The listing builds one solid part. Answer for the finished solid, in the listing's coordinates (mm). A direction names the side the tool comes from. Coordinates: 2 decimals unless noted, no trailing zeros. Order: outer loops, then holes, each group sorted by start corner. A loop starts at its lowest first (then second) coordinate and runs counter-clockwise, first axis right, second up. Notation, with made-up numbers: (-6, -4) - (43, -4) arc R11 ccw to (43, 16) - close; hole circle Ø3 at (-28, 54.25). An arc over 180 degrees is marked (long way). Use one line per item in the form item = value. Start each with the question number.
Item 1: Consider line 1 along X through (y, z) = (-66.3, 0); line 2 along X through (y, z) = (-68.85, 0); line 3 along X through (y, z) = (-64.5, 0). Determine where each line is inside the solid, lowest interval first. Write a range as [from, to].
Item 2: The mould has two halves that part along Z. Classify faces 1 (the flat face through (13, -66.8, -3)), 2 (the cylindrical face through (21.07, -64.93, -5.5)), 3 (the flat face through (-22.5, -65, 0)), 4 (the flat face through (2, 0, -5)): released by +Z, released by -Z, zero draft, split by the parting line, or undercut.
Item 3: Each of these flat-tipped pins is pushed along its axis until it touches: pin 1 Ø4.5 at (x, y) = (1, 0.5) entering from +Z; pin 2 Ø2 at (x, z) = (6.5, 0) entering from -Y; pin 3 Ø3 at (x, z) = (-5, -1) entering from +Y. Where does it stop, or does it pass through?
Item 4: Section A-A, the plane y = -58 is taken. Write down the section's boundary in (x, z).
Item 5: A tool of negligible diameter and unlimited length cuts with its end or side. For faces 5 (the cylindrical face through (-7.493, 0.33, -0.563)), 6 (the flat face through (-20, -60, -3)), 7 (the cylindrical face through (-21, -65.07, 5.57)), 8 (the cylindrical face through (9.63, -63.35, -1.19)), 9 (the cylindrical face through (-6.399, -67.465, 1.908)), from which of +Z, -Z, +X, -X, +Y, -Y can it reach the whole face along a straight path? Write none if from no direction.
from build123d import *

# Parameters (mm, degrees)
SKETCH_1_R                = 15
SKETCH_1_R_2              = 0.5
EXTRUDE_1_DEPTH           = 7
CUT_EXTRUDE_START         = -12
SKETCH_2_R                = 7.5
SKETCH_2_R_2              = 0.5
CUT_EXTRUDE_1_DEPTH       = 12
CHAMFER_1_SIZE            = 3
EXTRUDE_2_DEPTH           = 7
CUT_EXTRUDE_2_DEPTH       = 5
FILLET_1_R                = 5
MM_1_D                    = 4
MM_1_DEPTH                = 5
MM_1_TIP                  = 1.201721238
HOLE_WIZARD_1_D           = 6.4
HOLE_WIZARD_1_DEPTH       = 10
HOLE_WIZARD_1_CBORE_D     = 11
HOLE_WIZARD_1_CBORE_DEPTH = 6.8


with BuildPart() as part:
    # 草图1 → 凸台-拉伸1 (new, symmetric)
    with BuildSketch(Plane.XY):
        Circle(SKETCH_1_R)
        Circle(SKETCH_1_R_2, mode=Mode.SUBTRACT)
    extrude(amount=EXTRUDE_1_DEPTH, both=True)

    # 草图2 → 切除-拉伸1 (cut)
    with BuildSketch(Plane.XY.offset(7).offset(CUT_EXTRUDE_START)):
        Circle(SKETCH_2_R)
        Circle(SKETCH_2_R_2, mode=Mode.SUBTRACT)
    extrude(amount=CUT_EXTRUDE_1_DEPTH, mode=Mode.SUBTRACT)

    # 倒角1
    chamfer_1_edges = [part.edges().sort_by_distance(p)[0] for p in [
        (-7.5, 0, 7),
    ]]
    chamfer(chamfer_1_edges, length=CHAMFER_1_SIZE)

    # 草图3 → 凸台-拉伸2 (add, symmetric)
    with BuildSketch(Plane.XY):
        with BuildLine():
            Line((-22.5, -60), (-22.5, -70))
            Line((-22.5, -70), (22.5, -70))
            Line((22.5, -70), (22.5, -60))
            Line((22.5, -60), (9, -60))
            Line((9, -60), (9, -12))
            ThreePointArc((9, -12), (0, -15), (-9, -12))
            Line((-9, -12), (-9, -60))
            Line((-9, -60), (-22.5, -60))
        make_face()
    extrude(amount=EXTRUDE_2_DEPTH, both=True)

    # 草图4 → 切除-拉伸2 (cut)
    with BuildSketch(Plane.XZ.offset(70)):
        with BuildLine():
            Line((6, 2), (8, 2))
            ThreePointArc((8, 2), (10, 0), (8, -2))
            Line((8, -2), (6, -2))
            ThreePointArc((6, -2), (4, 0), (6, 2))
        make_face()
    extrude(amount=-CUT_EXTRUDE_2_DEPTH, mode=Mode.SUBTRACT)

    # 圆角1
    fillet_1_edges = [part.edges().sort_by_distance(p)[0] for p in [
        (-22.5, -65, -7),
        (22.5, -65, 7),
        (-22.5, -65, 7),
        (22.5, -65, -7),
    ]]
    fillet(fillet_1_edges, radius=FILLET_1_R)

    # 大小mm 暗销孔1
    with Locations(Plane(origin=(-7, -70, 0), x_dir=(0, 0, -1), z_dir=(0, -1, 0))):
        with Locations((0, 0)):
            Hole(MM_1_D / 2, depth=MM_1_DEPTH)
            with Locations((0, 0, -(MM_1_DEPTH + MM_1_TIP / 2))):  # 118° drill point
                Cone(0, MM_1_D / 2, MM_1_TIP, mode=Mode.SUBTRACT)

    # 打孔尺寸(%根据)内六角圆柱头螺钉的类型1
    with Locations(Plane(origin=(-15, -60, 0), x_dir=(0, 0, 1), z_dir=(0, 1, 0))):
        with Locations((0, 0), (0, 30)):
            CounterBoreHole(HOLE_WIZARD_1_D / 2, HOLE_WIZARD_1_CBORE_D / 2, HOLE_WIZARD_1_CBORE_DEPTH, depth=HOLE_WIZARD_1_DEPTH)


solid = part.part
Response:
q1.line_1 = [-22.5, -20.5], [-9.5, -9], [-5, 4], [20.5, 22.5]
q1.line_2 = [-22.5, -18.2], [-11.8, -9], [-5, 4], [10, 11.8], [18.2, 22.5]
q1.line_3 = [-22.5, -20.5], [-9.5, -8.17], [-5.83, 9.5], [20.5, 22.5]
q2.face_1 = undercut
q2.face_2 = released by -Z
q2.face_3 = zero draft
q2.face_4 = released by +Z
q3.pin_1 = -5
q3.pin_2 = -65
q3.pin_3 = 14.59
q4.outline = (-9, -7) - (9, -7) - (9, 7) - (-9, 7) - close
q5.face_5 = +Z
q5.face_6 = +Z, -Z, -X
q5.face_7 = +Z, -X, +Y, -Y
q5.face_8 = none
q5.face_9 = -Y
